Verification items for the finished model (mm, model axes). A direction names the side the tool comes from. Give positions to 0.01 mm unless a question says otherwise; leave off trailing zeros. Write each loop counter-clockwise with the first axis right and the second up, starting at its lowest first coordinate (ties: lowest second). Pieces come first, ordered by that corner, then holes. Notation, with made-up numbers: M 60.25,34.5 L 82.25,34.5 A21 cw 82.25,64.5 Z; hole C 12,-31.5 d10. An arc over 180 degrees is marked long. Write item = value, one per line.
from build123d import *

# Parameters (mm, degrees)
ESQUISSE1_W             = 60
ESQUISSE1_H             = 80
BOSS_EXTRU_1_DEPTH      = 10
ESQUISSE3_W             = 15
ESQUISSE3_H             = 45
BOSS_EXTRU_2_DEPTH      = 10
ESQUISSE2_R             = 2.5
ENL_V_MAT_EXTRU_1_DEPTH = 10
CHANFREIN1_SIZE         = 5


with BuildPart() as part:
    # Esquisse1 → Boss.-Extru.1 (new body)
    with BuildSketch(Plane.XY):
        with Locations((30, 40)):
            Rectangle(ESQUISSE1_W, ESQUISSE1_H)
    extrude(amount=BOSS_EXTRU_1_DEPTH)

    # Esquisse3 → Boss.-Extru.2 (add)
    with BuildSketch(Plane.XY.offset(10)):
        with Locations((-7.5, 22.5)):
            Rectangle(ESQUISSE3_W, ESQUISSE3_H)
        with Locations((67.5, 22.5)):
            Rectangle(ESQUISSE3_W, ESQUISSE3_H)
    extrude(amount=-BOSS_EXTRU_2_DEPTH)

    # Esquisse2 → Enlèv. mat.-Extru.1 (cut)
    with BuildSketch(Plane.XY.offset(10)):
        with Locations((45, 75)):
            Circle(ESQUISSE2_R)
        with Locations((30, 75)):
            Circle(ESQUISSE2_R)
        with Locations(Location((15, 75, 0), (0, 0, 180))):
            Circle(ESQUISSE2_R)
        with Locations((-7.5, 22.5)):
            Circle(ESQUISSE2_R)
        with Locations((-7.5, 37.5)):
            Circle(ESQUISSE2_R)
        with Locations(Location((-7.5, 7.5, 0), (0, 0, 180))):
            Circle(ESQUISSE2_R)
        with Locations((67.5, 7.5)):
            Circle(ESQUISSE2_R)
        with Locations(Location((67.5, 37.5, 0), (0, 0, 180))):
            Circle(ESQUISSE2_R)
        with Locations(Location((67.5, 22.5, 0), (0, 0, 180))):
            Circle(ESQUISSE2_R)
    extrude(amount=-ENL_V_MAT_EXTRU_1_DEPTH, mode=Mode.SUBTRACT)

    # Chanfrein1
    chanfrein1_edges = [part.edges().sort_by_distance(p)[0] for p in [
        (-15, 0, 5),
        (75, 0, 5),
    ]]
    chamfer(chanfrein1_edges, length=CHANFREIN1_SIZE)


solid = part.part
1) Cross-section at A-A on x = 30. Record the boundary of the cut face in (y, z).
From the geometry:
outline = M 0,0 L 72.5,0 L 72.5,10 L 0,10 Z; M 77.5,0 L 80,0 L 80,10 L 77.5,10 Z
2) Cross-section at B-B on y = 22.5. Record the boundary of the cut face in (x, z), plus the area to 3 significant figures.
From the geometry:
outline = M -15,0 L -10,0 L -10,10 L -15,10 Z; M -5,0 L 65,0 L 65,10 L -5,10 Z; M 70,0 L 75,0 L 75,10 L 70,10 Z
area = 800 mm^2
3) Draft check along X on faces 4 (the flat face through (29, 41, 10)), 5 (the flat face through (-15, 25, 5)), 6 (the cylindrical face through (-8.04, 35.06, 5.07)). Enter one of: +X half, -X half, draft (parallel to the pull), parting line (faces both ways), or undercut.
From the geometry:
face_4 = draft
face_5 = -X half
face_6 = undercut
4) Material ranges on probe 1 along Y at (x, z) = (-7.5, 4.75); probe 2 along Y at (x, z) = (69.5, 4); probe 3 along X at (y, z) = (23, 5.25), recorded low to high. Write a range as from..to.
From the geometry:
probe_1 = 0..5, 10..20, 25..35, 40..45
probe_2 = 0..6, 9..21, 24..36, 39..45
probe_3 = -15..-9.95, -5.05..65.05, 69.95..75
5) Tool access check on faces 1 (the flat face through (60, 62, 5)), 2 (the cylindrical face through (-7.83, 24.98, 5.07)), 3 (the flat face through (-8, 45, 5)). Record the directions out of +Z, -Z, +X, -X, +Y, -Y that give a thin tool (end or side, any length) a straight path to the whole face; none if there is none.
From the geometry:
face_1 = +Z, -Z, +X, +Y
face_2 = +Z, -Z
face_3 = +Z, -Z, -X, +Y
6) Cross-section at D-D on z = 8.5. Count the separate pieces of the cut face and the enclosed holes in it, plus the area to 3 significant figures.
From the geometry:
separate_pieces = 1
enclosed_holes = 9
area = 5,950 mm^2
7) Cross-section at C-C on y = 75. Record the boundary of the cut face in (x, z), plus the area to 3 significant figures.
From the geometry:
outline = M 0,0 L 12.5,0 L 12.5,10 L 0,10 Z; M 17.5,0 L 27.5,0 L 27.5,10 L 17.5,10 Z; M 32.5,0 L 42.5,0 L 42.5,10 L 32.5,10 Z; M 47.5,0 L 60,0 L 60,10 L 47.5,10 Z
area = 450 mm^2
8) Depth check by flat-ended pin: P1, Ø3, axis at x = 68, z = 4.5, coming from the +Y side; P2, Ø1.5, axis at y = 47.5, z = 3, coming from the -X side. Enter the tip coordinate at first touch or a pass-through.
From the geometry:
P1 = 45
P2 = 0
